Build history of the part. All positions in model axes, mm. Round coordinates to 2 decimals unless told otherwise and drop trailing zeros. Write each loop counter-clockwise with the first axis right and the second up, starting at its lowest first coordinate (ties: lowest second). Pieces come first, ordered by that corner, then holes. Notation, with made-up numbers: (-7, 13) -> (17, 13) arc R9 ccw to (17, 30) -> close; hole circle Ø1 at (-6, 80.5). An arc over 180 degrees is marked (long way). Return JSON: item names as keys, results as strings.
from build123d import *

# Parameters (mm, degrees)
SKETCH1_R              = 6
SKETCH1_R_2            = 3
BOSS_EXTRUDE1_DEPTH    = 8
CUT_EXTRUDE1_START     = -6.000000101
CUT_EXTRUDE1_OUTLINE_R = 1
CUT_EXTRUDE1_DEPTH     = 12.000000201


# Read off the part's stored shape, not the designer's step: Cut-Extrude1
with BuildPart() as part:
    # Sketch1 → Boss-Extrude1 (new body)
    with BuildSketch(Plane(origin=(0, 0, 0), x_dir=(1, 0, 0), z_dir=(0, 1, 0))):
        with Locations(Location((0, 0, 0), (0, 0, 270))):
            Circle(SKETCH1_R)
        with Locations(Location((0, 0, 0), (0, 0, 270))):
            Circle(SKETCH1_R_2, mode=Mode.SUBTRACT)
    extrude(amount=BOSS_EXTRUDE1_DEPTH)

    # Cut-Extrude1 outline → Cut-Extrude1 (cut)
    with BuildSketch(Plane.XY.offset(CUT_EXTRUDE1_START)):
        with Locations((0, 1.5)):
            Circle(CUT_EXTRUDE1_OUTLINE_R)
        with Locations((0, 5.5)):
            Circle(CUT_EXTRUDE1_OUTLINE_R)
    extrude(amount=CUT_EXTRUDE1_DEPTH, mode=Mode.SUBTRACT)


solid = part.part
Q1. Saw through at A-A on x = 0. List the corners of the cut face in (y, z).
Verdict:
{"outline": "(0, -6) -> (0.5, -6) -> (0.5, -3) -> (0, -3) -> close; (0, 3) -> (0.5, 3) -> (0.5, 6) -> (0, 6) -> close; (2.5, -6) -> (4.5, -6) -> (4.5, -3) -> (2.5, -3) -> close; (2.5, 3) -> (4.5, 3) -> (4.5, 6) -> (2.5, 6) -> close; (6.5, -6) -> (8, -6) -> (8, -3) -> (6.5, -3) -> close; (6.5, 3) -> (8, 3) -> (8, 6) -> (6.5, 6) -> close"}
Q2. Two-plate mould, pull along X, no slides. Class faces 1 (the cylindrical face through (0.954, 5.8, 4.392)), 2 (the cylindrical face through (-1.15, 3.94, 2.77)), 3 (the cylindrical face through (1.802, 3.944, 5.723)), 4 (the flat face through (3, 0, 1)): +X half, -X half, draft (parallel to the pull), parting line (faces both ways), or undercut.
Verdict:
{"face 1": "undercut", "face 2": "undercut", "face 3": "parting line", "face 4": "draft"}
Q3. Saw through at C-C on y = 1.5. List the corners of the cut face in (x, z).
Verdict:
{"outline": "(-1, -5.92) -> (-1, -2.83) arc R3 cw to (-1, 2.83) -> (-1, 5.92) arc R6 ccw to start; (1, -5.92) arc R6 ccw to (1, 5.92) -> (1, 2.83) arc R3 cw to (1, -2.83) -> close"}
Q4. Wall check: L1, parallel to Y at x = 0, z = 3.7; L2, parallel to X at y = 4.5, z = 0. Give the ranges that are in metal, low to high.
Verdict:
{"L1": "y = 0 to 0.5, 2.5 to 4.5, 6.5 to 8", "L2": "x = -6 to -3, 3 to 6"}
Q5. Saw through at B-B on z = 0. List the corners of the cut face in (x, y), then the cut area to 3 significant figures.
Verdict:
{"outline": "(-6, 0) -> (-3, 0) -> (-3, 8) -> (-6, 8) -> close; (3, 0) -> (6, 0) -> (6, 8) -> (3, 8) -> close", "area": "48.0 mm²"}
Q6. Pin check, flat tips, straight feed: pin 1 Ø2 at (y, z) = (2, -3) entering from +X; pin 2 Ø1 at (x, y) = (1, 1) entering from +Z; pin 3 Ø1.2 at (x, y) = (0, 5.5) entering from +Z. Stop position of each tip, or through.
Verdict:
{"pin 1": "stops at x = 5.66", "pin 2": "stops at z = 5.97", "pin 3": "passes through"}
Q7. Saw through at D-D on y = 3.5. List the corners of the cut face in (x, z), then the cut area to 3 significant figures.
Verdict:
{"outline": "circle Ø12 at (0, 0); hole circle Ø6 at (0, 0)", "area": "84.8 mm²"}
